```python
from build123d import *

# Parameters (mm, degrees)
F0_R     = 34.925
F1_DEPTH = 6.35
F2_SIZE  = 2.54
F3_R     = 12.7
F3_R_2   = 7.14375
F4_DEPTH = 19.05


with BuildPart() as f1:
    # F0 (on Front) → F1 (new body)
    with BuildSketch(Plane.XZ):
        Circle(F0_R)
    extrude(amount=F1_DEPTH)

    # F2
    f2_edges = [f1.edges().sort_by_distance(p)[0] for p in [
        (-34.925, -6.35, 0),
    ]]
    chamfer(f2_edges, length=F2_SIZE)

    # F3 (on face) → F4 (join)
    with BuildSketch(Plane(origin=(0, 0, 0), x_dir=(-1, 0, 0), z_dir=(0, 1, 0))):
        Circle(F3_R)
        Circle(F3_R_2, mode=Mode.SUBTRACT)
    extrude(amount=F4_DEPTH)


solid = f1.part
```
For this review, take the finished solid that the model builds, in its own axes (mm). A direction names the side the tool comes from. Round coordinates to 2 decimals unless told otherwise and drop trailing zeros. Order: outer loops, then holes, each group sorted by start corner. A loop starts at its lowest first (then second) coordinate and runs counter-clockwise, first axis right, second up. Notation, with made-up numbers: (75, -33) -> (98, -33) arc R8 ccw to (98, -26) -> close; hole circle Ø7 at (10.25, 61.25). An arc over 180 degrees is marked (long way). Use a Markdown table: item, result.
Item 1: Draft analysis for pull direction Z (two halves, no side actions). For faces 1 (the cylindrical face through (7.137, 9.392, 0.314)), 2 (the conical face through (-4.23, -6.23, 32.23)), 3 (the flat face through (15, 0, 0)), state which applies: +Z half, -Z half, draft (parallel to the pull), parting line (faces both ways), or undercut.
Resolved:
| item | result |
|---|---|
| face 1 | undercut |
| face 2 | parting line |
| face 3 | draft |
Item 2: Take a section at A-A (z = 0). State the section outline as (x, y) points (3 decimals), plus the area to 3 significant figures.
Resolved:
| item | result |
|---|---|
| outline | (-34.925, -3.81) -> (-32.385, -6.35) -> (32.385, -6.35) -> (34.925, -3.81) -> (34.925, 0) -> (12.7, 0) -> (12.7, 19.05) -> (7.144, 19.05) -> (7.144, 0) -> (-7.144, 0) -> (-7.144, 19.05) -> (-12.7, 19.05) -> (-12.7, 0) -> (-34.925, 0) -> close |
| area | 649 mm² |
Item 3: Take a section at C-C (y = 16.75). State the section outline as (x, z) points, plus the area to 3 significant figures.
Resolved:
| item | result |
|---|---|
| outline | circle Ø25.4 at (0, 0); hole circle Ø14.29 at (0, 0) |
| area | 346 mm² |
Item 4: Machinability: for faces 4 (the flat face through (0, -6.35, 0)), 5 (the cylindrical face through (2.75, 9.39, -12.4)), which of the approach directions +Z, -Z, +X, -X, +Y, -Y give a long, thin tool a straight path to every point of the face, cutting with its end or side? Answer none if there is none.
Resolved:
| item | result |
|---|---|
| face 4 | +Z, -Z, +X, -X, -Y |
| face 5 | +Y |
Item 5: Take a section at D-D (y = -2.75). State the section outline as (x, z) points (3 decimals), plus the area to 3 significant figures.
Resolved:
| item | result |
|---|---|
| outline | circle Ø69.85 at (0, 0) |
| area | 3,830 mm² |
Item 6: Take a section at B-B (x = 0). State the section outline as (y, z) points (3 decimals).
Resolved:
| item | result |
|---|---|
| outline | (-6.35, -32.385) -> (-3.81, -34.925) -> (0, -34.925) -> (0, -12.7) -> (19.05, -12.7) -> (19.05, -7.144) -> (0, -7.144) -> (0, 7.144) -> (19.05, 7.144) -> (19.05, 12.7) -> (0, 12.7) -> (0, 34.925) -> (-3.81, 34.925) -> (-6.35, 32.385) -> close |
Item 7: For pin 1 (1.5 mm diameter, centred on x = -3, y = 9, fed in from -Z); pin 2 (4.5 mm diameter, centred on x = -1.5, z = 2.5, fed in from +Y); pin 3 (10 mm diameter, centred on x = 4, y = 9, fed in from +Z), all flat-tipped, find the tip position at first contact; note any pin that passes through.
Resolved:
| item | result |
|---|---|
| pin 1 | stops at z = -12.5 |
| pin 2 | stops at y = 0 |
| pin 3 | stops at z = 12.7 |
Item 8: For line 1 along Z through (x, y) = (0, 13.75); line 2 along Y through (x, z) = (16, -27.5); line 3 along Z through (x, y) = (-2, 10), list the stretches that pass through material, from the lowest coordinate up. Write a range as [from, to].
Resolved:
| item | result |
|---|---|
| line 1 | z = [-12.7, -7.14], [7.14, 12.7] |
| line 2 | y = [-6.35, 0] |
| line 3 | z = [-12.54, -6.86], [6.86, 12.54] |
